Input: part model. Units: mm. Frame: model coordinates. Give positions to 0.01 mm unless a question says otherwise; leave off trailing zeros. Write each loop counter-clockwise with the first axis right and the second up, starting at its lowest first coordinate (ties: lowest second). Pieces come first, ordered by that corner, then holes. Notation, with made-up numbers: (62.25, 83) - (115.25, 83) arc R31 ccw to (115.25, 117) - close; hole circle Ø4 at (-17.5, 39.5). An arc over 180 degrees is marked (long way). Use a Markdown table: item, result. Add a question column.
1. Material intervals for probe 1 along Y at (x, z) = (0, 344.5); probe 2 along Z at (x, y) = (4.5, 4.75); probe 3 along X at (y, z) = (-5.75, 127), sorted ascending.
2. Section query A-A, the plane x = 0. Return loops of the section in (y, z), plus the area to 3 significant figures.
3. Section query B-B, the plane z = 72. Return loops of the section in (x, y) (1 decimal), plus the area to 3 significant figures.
4. Pin query (flat end, axial travel): pin 1 (2.5 mm diameter, centred on y = -1.5, z = 175, fed in from -X); pin 2 (12 mm diameter, centred on x = 4, z = 289, fed in from -Y); pin 3 (0.8 mm diameter, centred on y = -2, z = 211.5, fed in from -X); pin 4 (8 mm diameter, centred on x = -7.5, z = 139, fed in from -Y). Return the tip coordinate at first contact, or that it passes through.
```python
from build123d import *

# Parameters (mm, degrees)
SKETCH1_R               = 10.4275
BOSS_EXTRUDE1_DEPTH     = 390
SKETCH2_R               = 7.112
CUT_EXTRUDE1_DEPTH      = 141.75
CUT_EXTRUDE2_START      = -141.75
SKETCH3_R               = 7.112
CUT_EXTRUDE2_DEPTH      = 141.75
CUT_EXTRUDE3_DEPTH      = 20
CUT_EXTRUDE3_DEPTH_BACK = 20
SKETCH4_W               = 2.8
SKETCH4_H               = 97.6
CUT_EXTRUDE4_DEPTH      = 20
LPATTERN1_COUNT         = 14
LPATTERN1_PITCH         = 6.7
SKETCH6_W               = 24.776384874
SKETCH6_H               = 25.11648024
CUT_EXTRUDE5_DEPTH      = 8.25
SKETCH7_W               = 32.905320966
SKETCH7_H               = 32.372251486
CUT_EXTRUDE6_DEPTH      = 8.25


with BuildPart() as part:
    # Sketch1 → Boss-Extrude1 (new body)
    with BuildSketch(Plane.XY):
        Circle(SKETCH1_R)
    extrude(amount=BOSS_EXTRUDE1_DEPTH)

    # Sketch2 → Cut-Extrude1 (cut)
    with BuildSketch(Plane(origin=(0, 0, 0), x_dir=(-1, 0, 0), z_dir=(0, 0, -1))):
        Circle(SKETCH2_R)
    extrude(amount=-CUT_EXTRUDE1_DEPTH, mode=Mode.SUBTRACT)

    # Sketch3 → Cut-Extrude2 (cut)
    with BuildSketch(Plane.XY.offset(390).offset(CUT_EXTRUDE2_START)):
        with Locations(Location((0, 0, 0), (0, 0, 180))):
            Circle(SKETCH3_R)
    extrude(amount=CUT_EXTRUDE2_DEPTH, mode=Mode.SUBTRACT)

    # Sketch4 → Cut-Extrude3 (cut, two sides: drawn at the far end of the back side and taken through both)
    with BuildSketch(Plane(origin=(0, 0, 0), x_dir=(1, 0, 0), z_dir=(0, 1, 0)).offset(-CUT_EXTRUDE3_DEPTH_BACK)):
        Polygon((6.189444989, -239.775), (6.189444989, -150.245179393), (10.438224829, -142.247476164), (10.438224829, -247.772703229), align=None)
        with Locations((-9.0275, -195.025)):
            Rectangle(SKETCH4_W, SKETCH4_H)
    extrude(amount=CUT_EXTRUDE3_DEPTH + CUT_EXTRUDE3_DEPTH_BACK, mode=Mode.SUBTRACT)

    # Sketch5 → Cut-Extrude4 (cut, symmetric)
    with BuildSketch(Plane(origin=(0, 0, 0), x_dir=(1, 0, 0), z_dir=(0, 1, 0))):
        Polygon((-3.4275, -152.275), (-3.4275, -150.675), (-7.6275, -149.175), (-7.6275, -153.775), align=None)
    cut_extrude4 = extrude(amount=CUT_EXTRUDE4_DEPTH, both=True, mode=Mode.SUBTRACT)

    # LPattern1: Cut-Extrude4 ×14
    with Locations(*[(0, 0, i * LPATTERN1_PITCH) for i in range(1, LPATTERN1_COUNT)]):
        add(cut_extrude4, mode=Mode.SUBTRACT)

    # Sketch6 → Cut-Extrude5 (cut)
    with BuildSketch(Plane.XY.offset(390)):
        Rectangle(SKETCH6_W, SKETCH6_H)
    extrude(amount=-CUT_EXTRUDE5_DEPTH, mode=Mode.SUBTRACT)

    # Sketch7 → Cut-Extrude6 (cut)
    with BuildSketch(Plane(origin=(0, 0, 0), x_dir=(-1, 0, 0), z_dir=(0, 0, -1))):
        Rectangle(SKETCH7_W, SKETCH7_H)
    extrude(amount=-CUT_EXTRUDE6_DEPTH, mode=Mode.SUBTRACT)


solid = part.part
```
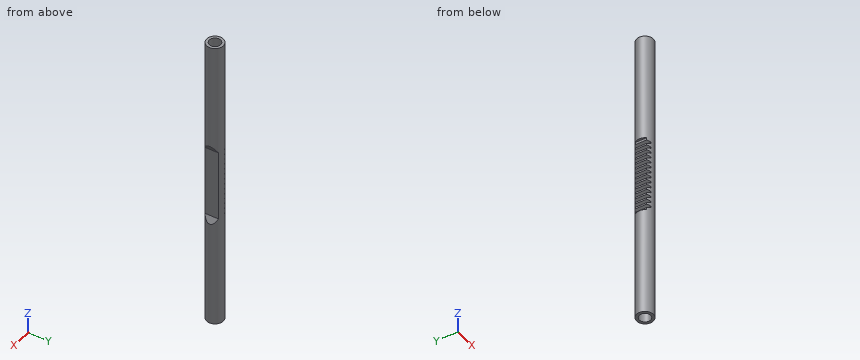
Result sheet:
| question | item | result |
|---|---|---|
| 1 | probe 1 | y = -10.43 to -7.11, 7.11 to 10.43 |
| 1 | probe 2 | z = 141.75 to 248.25 |
| 1 | probe 3 | x = -8.7 to -4.19, 4.19 to 8.7 |
| 2 | outline | (-10.43, 8.25) - (-7.11, 8.25) - (-7.11, 141.75) - (7.11, 141.75) - (7.11, 8.25) - (10.43, 8.25) - (10.43, 381.75) - (7.11, 381.75) - (7.11, 248.25) - (-7.11, 248.25) - (-7.11, 381.75) - (-10.43, 381.75) - close |
| 2 | area | 3,990 mm² |
| 3 | outline | circle Ø20.9 at (0, 0); hole circle Ø14.2 at (0, 0) |
| 3 | area | 183 mm² |
| 4 | pin 1 | stops at x = -7.63 |
| 4 | pin 2 | stops at y = -10.43 |
| 4 | pin 3 | stops at x = -3.43 |
| 4 | pin 4 | stops at y = -9.82 |
